Design review of the part shown in the three views and the two pictorial views. Dimensions are in mm from the part's minimum x, y and z. Coordinates: 2 decimals unless noted, no trailing zeros. Order: outer loops, then holes, each group sorted by start corner. A loop starts at its lowest first (then second) coordinate and runs counter-clockwise, first axis right, second up. Notation, with made-up numbers: (-23, -10.5) -> (5, -10.5) arc R25 ccw to (5, 23.5) -> close; hole circle Ø1 at (29, 66.5). An arc over 180 degrees is marked (long way). Write item = value, one per line. Start each with the question number.
1) Wall thickness on probe 1 along Y at (x, z) = (339.5, 42.5); probe 2 along Z at (x, y) = (34.5, 322.5); probe 3 along X at (y, z) = (47, 157): over which ranges is each line inside the solid? List them lowest first. Write a range as [from, to].
2) Consider section D-D on y = 332. Give the boundary of the cut face in (x, z), and give its area (3 significant figures).
3) Consider section A-A on z = 239. Give the boundary of the cut face in (x, y).
4) Insertion check: pin 1 Ø2 at (x, y) = (292.5, 325.5) entering from -Z; pin 2 Ø8 at (x, z) = (51, 206.5) entering from +Y; pin 3 Ø1 at (y, z) = (78.5, 51.5) entering from -X. Each pin has a flat end and moves straight along its axis. Give the tip position at first contact, or say it passes through.
5) Consider section B-B on y = 54.5. Give the boundary of the cut face in (x, z), and give its area (3 significant figures).
6) Draft analysis for pull direction X (two halves, no side actions). For the marked faces 1 and 2, state which applies: +X half, -X half, draft (parallel to the pull), parting line (faces both ways), or undercut.
7) Consider section C-C on x = 281. Give the boundary of the cut face in (y, z), and give its area (3 significant figures).
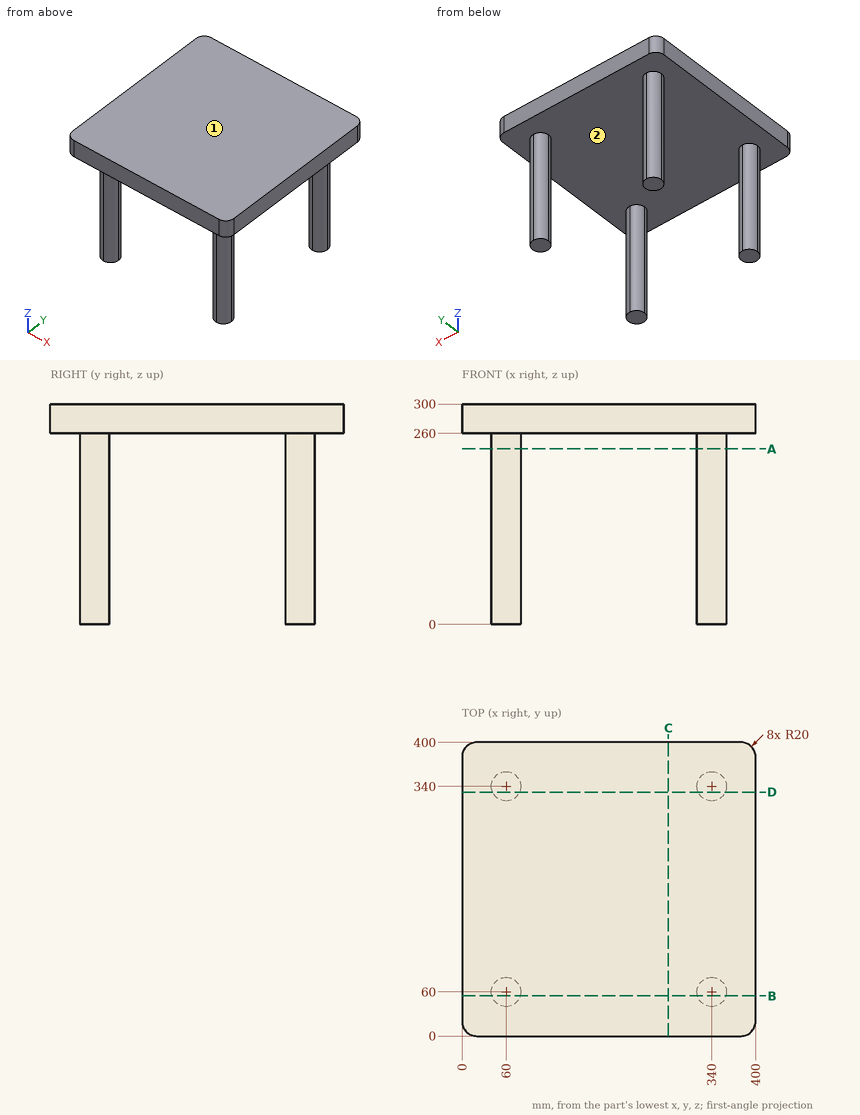
Answer sheet:
q1.probe_1 = [40.01, 79.99], [320.01, 359.99]
q1.probe_2 = [260, 300]
q1.probe_3 = [44.8, 75.2], [324.8, 355.2]
q2.outline = (0, 260) -> (41.67, 260) -> (41.67, 0) -> (78.33, 0) -> (78.33, 260) -> (321.67, 260) -> (321.67, 0) -> (358.33, 0) -> (358.33, 260) -> (400, 260) -> (400, 300) -> (0, 300) -> close
q2.area = 35,100 mm2
q3.outline = (40, 60) arc R20 ccw to (60, 40) arc R20 ccw to (80, 60) arc R20 ccw to (60, 80) arc R20 ccw to start; (40, 340) arc R20 ccw to (60, 320) arc R20 ccw to (80, 340) arc R20 ccw to (60, 360) arc R20 ccw to start; (320, 60) arc R20 ccw to (340, 40) arc R20 ccw to (360, 60) arc R20 ccw to (340, 80) arc R20 ccw to start; (320, 340) arc R20 ccw to (340, 320) arc R20 ccw to (360, 340) arc R20 ccw to (340, 360) arc R20 ccw to start
q4.pin_1 = 260
q4.pin_2 = 359.36
q4.pin_3 = 51.28
q5.outline = (0, 260) -> (40.77, 260) -> (40.77, 0) -> (79.23, 0) -> (79.23, 260) -> (320.77, 260) -> (320.77, 0) -> (359.23, 0) -> (359.23, 260) -> (400, 260) -> (400, 300) -> (0, 300) -> close
q5.area = 36,000 mm2
q6.face_1 = draft
q6.face_2 = undercut
q7.outline = (0, 260) -> (400, 260) -> (400, 300) -> (0, 300) -> close
q7.area = 16,000 mm2
